Read the model definition and answer for the solid it produces. Units are mm, in the model's axes. Face numbers are marked on the shaded views. A direction names the side the tool comes from. Coordinates: 2 decimals unless noted, no trailing zeros. Loops run counter-clockwise (first coordinate to the right, second up) from the corner with the lowest first, then second, coordinate; pieces in that order, holes last. Notation, with made-up numbers: (-25.5, 23) - (28.5, 23) arc R24 cw to (28.5, 33) - close; hole circle Ø5 at (-3, 0.25). An arc over 180 degrees is marked (long way). Use CSV: the item, a comma, the result in double quotes.
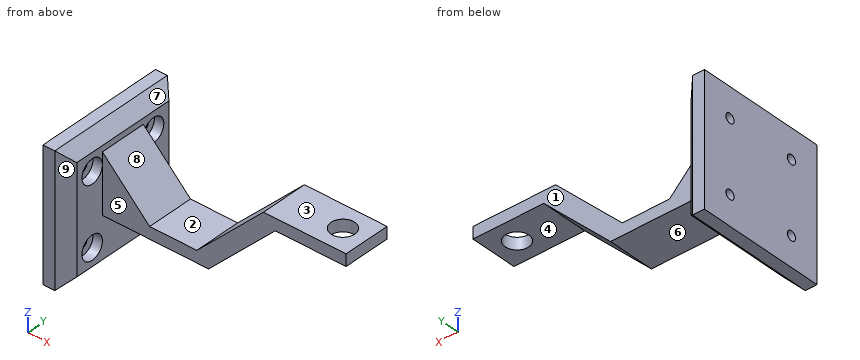
```python
from build123d import *

# Parameters (mm, degrees)
SKETCH1_W           = 20
SKETCH1_H           = 20
SKETCH1_R           = 5
BOSS_EXTRUDE1_DEPTH = 5
SKETCH2_W           = 5
SKETCH2_H           = 20
BOSS_EXTRUDE2_DEPTH = 15
BOSS_EXTRUDE3_DEPTH = 20
SKETCH4_W           = 55
SKETCH4_H           = 55
BOSS_EXTRUDE4_DEPTH = 10
CHAMFER1_SIZE       = 20
CHAMFER2_SIZE       = 5
SKETCH5_R           = 2
CUT_EXTRUDE1_DEPTH  = 119.333988749
SKETCH6_R           = 5
SKETCH6_R_2         = 2
CUT_EXTRUDE2_DEPTH  = 4


with BuildPart() as part:
    # Sketch1 → Boss-Extrude1 (new body)
    with BuildSketch(Plane.XY):
        Rectangle(SKETCH1_W, SKETCH1_H)
        Circle(SKETCH1_R, mode=Mode.SUBTRACT)
    extrude(amount=BOSS_EXTRUDE1_DEPTH)

    # Sketch2 → Boss-Extrude2 (add)
    with BuildSketch(Plane.ZY.offset(10)):
        with Locations((2.5, 0)):
            Rectangle(SKETCH2_W, SKETCH2_H)
    extrude(amount=BOSS_EXTRUDE2_DEPTH)

    # Sketch3 → Boss-Extrude3 (add)
    with BuildSketch(Plane.XZ.offset(10)):
        Polygon((-25, 0), (-25, 5), (-53.284271247, -23.284271247), (-48.284271247, -23.284271247), (-48.284271247, -28.284271247), (-20, 0), align=None)
        Polygon((-48.284271247, -28.284271247), (-53.284271247, -23.284271247), (-93.284271247, -23.284271247), (-93.284271247, -28.284271247), align=None)
        Polygon((-48.284271247, -23.284271247), (-53.284271247, -23.284271247), (-48.284271247, -28.284271247), align=None)
    extrude(amount=-BOSS_EXTRUDE3_DEPTH)

    # Sketch4 → Boss-Extrude4 (add)
    with BuildSketch(Plane.ZY.offset(93.284271247)):
        with Locations((-23.284271247, 0)):
            Rectangle(SKETCH4_W, SKETCH4_H)
    extrude(amount=BOSS_EXTRUDE4_DEPTH)

    # Chamfer1
    chamfer1_edges = [part.edges().sort_by_distance(p)[0] for p in [
        (-93.284271247, 0, -23.284271247),
    ]]
    chamfer(chamfer1_edges, length=CHAMFER1_SIZE)

    # Chamfer2
    chamfer2_edges = [part.edges().sort_by_distance(p)[0] for p in [
        (-93.284271247, 0, -50.784271247),
        (-93.284271247, -27.5, -23.284271247),
        (-93.284271247, 0, 4.215728753),
        (-93.284271247, 27.5, -23.284271247),
    ]]
    chamfer(chamfer2_edges, length=CHAMFER2_SIZE)

    # Sketch5 → Cut-Extrude1 (cut, through all)
    with BuildSketch(Plane(origin=(-93.284271247, 0, 0), x_dir=(0, 0, -1), z_dir=(1, 0, 0))):
        with Locations((38.284271247, 15)):
            Circle(SKETCH5_R)
        with Locations(Location((38.284271247, -15, 0), (0, 0, 180))):
            Circle(SKETCH5_R)
        with Locations((8.284271247, -15)):
            Circle(SKETCH5_R)
        with Locations(Location((8.284271247, 15, 0), (0, 0, 180))):
            Circle(SKETCH5_R)
    extrude(amount=-CUT_EXTRUDE1_DEPTH, mode=Mode.SUBTRACT)

    # Sketch6 → Cut-Extrude2 (cut)
    # profile 1 of 4: a face of its own
    with BuildSketch(Plane(origin=(-93.284271247, 0, 0), x_dir=(0, 0, -1), z_dir=(1, 0, 0))):
        with Locations((8.284271247, 15)):
            Circle(SKETCH6_R)
        with Locations((8.284271247, 15)):
            Circle(SKETCH6_R_2, mode=Mode.SUBTRACT)
    # profile 2 of 4: a face of its own
    with BuildSketch(Plane(origin=(-93.284271247, 0, 0), x_dir=(0, 0, -1), z_dir=(1, 0, 0))):
        with Locations((8.284271247, -15)):
            Circle(SKETCH6_R)
        with Locations((8.284271247, -15)):
            Circle(SKETCH6_R_2, mode=Mode.SUBTRACT)
    # profile 3 of 4: a face of its own
    with BuildSketch(Plane(origin=(-93.284271247, 0, 0), x_dir=(0, 0, -1), z_dir=(1, 0, 0))):
        with Locations((38.284271247, -15)):
            Circle(SKETCH6_R)
        with Locations((38.284271247, -15)):
            Circle(SKETCH6_R_2, mode=Mode.SUBTRACT)
    # profile 4 of 4: a face of its own
    with BuildSketch(Plane(origin=(-93.284271247, 0, 0), x_dir=(0, 0, -1), z_dir=(1, 0, 0))):
        with Locations((38.284271247, 15)):
            Circle(SKETCH6_R)
        with Locations((38.284271247, 15)):
            Circle(SKETCH6_R_2, mode=Mode.SUBTRACT)
    extrude(amount=-CUT_EXTRUDE2_DEPTH, mode=Mode.SUBTRACT)


solid = part.part
```
Q1. Given P1, Ø1.5, axis at x = -83, y = 9.5, coming from the -Z side; P2, Ø5, axis at y = -15, z = -9.5, coming from the +X side; P3, Ø22, axis at x = -64.5, y = 2.5, coming from the +Z side, each flat-ended and moving along its own axis, determine where each tip first touches the part or whether it passes through.
Reported:
P1,"stops at z = -28.28"
P2,"stops at x = -97.28"
P3,"stops at z = -21.07"
Q2. The part is cut by section C-C on y = 0. Determine the outline of the cut face in (x, z).
Reported:
outline,"(-103.28, -50.78) - (-98.28, -50.78) - (-93.28, -45.78) - (-93.28, -28.28) - (-48.28, -28.28) - (-20, 0) - (-5, 0) - (-5, 5) - (-25, 5) - (-53.28, -23.28) - (-73.28, -23.28) - (-93.28, -3.28) - (-93.28, -0.78) - (-98.28, 4.22) - (-103.28, 4.22) - close; (5, 0) - (10, 0) - (10, 5) - (5, 5) - close"
Q3. The part is cut by section B-B on x = 0. Determine the outline of the cut face in (y, z), and give its area (3 significant figures).
Reported:
outline,"(-10, 0) - (-5, 0) - (-5, 5) - (-10, 5) - close; (5, 0) - (10, 0) - (10, 5) - (5, 5) - close"
area,"50.0 mm²"
Q4. A tool of negligible diameter and unlimited length cuts with its end or side. For the marked faces 1, 2, 3, 4 and 5, from which of +Z, -Z, +X, -X, +Y, -Y can it reach the whole face along a straight path? Write none if from no direction.
Reported:
face 1,"+Z, -Z, +X, +Y"
face 2,"+Z, +Y, -Y"
face 3,"+Z, +X, -X, +Y, -Y"
face 4,"-Z, +X, +Y, -Y"
face 5,"+Z, -Z, +X, -Y"
Q5. The part is cut by section D-D on z = -26.5. Determine the outline of the cut face in (x, y), and give its area (3 significant figures).
Reported:
outline,"(-103.28, -27.5) - (-98.28, -27.5) - (-93.28, -22.5) - (-93.28, -10) - (-46.5, -10) - (-46.5, 10) - (-93.28, 10) - (-93.28, 22.5) - (-98.28, 27.5) - (-103.28, 27.5) - close"
area,"1,460 mm²"
Q6. For a pull along X with two mould halves and no side action, classify the marked faces 6, 7, 8 and 9 as +X half, -X half, draft (parallel to the pull), parting line (faces both ways), or undercut.
Reported:
face 6,"draft"
face 7,"undercut"
face 8,"undercut"
face 9,"+X half"
Q7. Find the intervals of material crossed by probe 1 along X at (y, z) = (-7, -34); probe 2 along X at (y, z) = (9, -3); probe 3 along Z at (x, y) = (-54.5, -4.5), in increasing order. Write a range as [from, to].
Reported:
probe 1,"x = [-103.28, -93.28]"
probe 2,"x = [-103.28, -93.28], [-33, -23]"
probe 3,"z = [-28.28, -23.28]"
Q8. The part is cut by section A-A on y = -15. Determine the outline of the cut face in (x, z), and give its area (3 significant figures).
Reported:
outline,"(-103.28, -50.78) - (-98.28, -50.78) - (-93.28, -45.78) - (-93.28, -43.28) - (-97.28, -43.28) - (-97.28, -40.28) - (-103.28, -40.28) - close; (-103.28, -36.28) - (-97.28, -36.28) - (-97.28, -33.28) - (-93.28, -33.28) - (-93.28, -13.28) - (-97.28, -13.28) - (-97.28, -10.28) - (-103.28, -10.28) - close; (-103.28, -6.28) - (-97.28, -6.28) - (-97.28, -3.28) - (-93.28, -3.28) - (-93.28, -0.78) - (-98.28, 4.22) - (-103.28, 4.22) - close"
area,"397 mm²"
